Source: CAD feature listing. Evaluate the final solid. Frame: model axes, mm. A direction names the side the tool comes from. Give positions to 0.01 mm unless a question says otherwise; leave off trailing zeros. Write each loop counter-clockwise with the first axis right and the second up, starting at its lowest first coordinate (ties: lowest second). Pieces come first, ordered by that corner, then holes. Notation, with made-up numbers: (21.5, -40) - (44.5, -40) arc R6 ccw to (44.5, -33) - close; hole circle Ø9 at (82.25, 86.5). An arc over 180 degrees is marked (long way). One line per question, with ' | ' between items. Start each with the question number.
(1) Access query for faces 4 (the flat face through (-87, -68, 3)), 5 (the flat face through (-99.875, -71, 3)), 6 (the flat face through (23, 1, 6)). Directions: +Z, -Z, +X, -X, +Y, -Y. A direction counts if a zero-diameter tool reaches every point of the face in a straight line with its end or side. Return the directions, or none.
(2) Pin query (flat end, axial travel): pin 1 (3 mm diameter, centred on y = 14, z = 3, fed in from -X). Return the tip coordinate at first contact, or that it passes through.
(3) Section A-A, the plane y = 0. Return loops of the section in (x, z), plus the area to 3 significant figures.
(4) Section B-B, the plane x = 103. Return loops of the section in (y, z), plus the area to 3 significant figures.
(5) Section C-C, the plane x = -103. Return loops of the section in (y, z), plus the area to 3 significant figures.
(6) Draft query along Y for faces 1 (the flat face through (-2, 84.5, 3)), 2 (the flat face through (-109.5, 76, 3)), 3 (the flat face through (-106.125, -71, 3)). Return one class per face: +Y half, -Y half, draft (parallel to the pull), parting line (faces both ways), or undercut.
(7) Section D-D, the plane y = -78. Return loops of the section in (x, z).
(8) Ray query, line 1 (X direction, y = 78, z = 4.2); line 2 (Y direction, x = 103, z = 3.2); line 3 (Y direction, x = -103, z = 2.75). Return the intervals inside material, ascending. Write a range as [from, to].
Autodesk Inventor part; units mm, degrees
sketch "Sketch1" plane through (0, 0, 0) normal (0, 0, 1) x (1, 0, 0)
  line L0 (-109.5, 84.5) -> (109.5, 84.5)
  line L1 (109.5, 84.5) -> (109.5, -84.5)
  line L2 (109.5, -84.5) -> (-109.5, -84.5)
  line L3 (-109.5, -84.5) -> (-109.5, 84.5)
  point P0 (0, 84.5)
  point P1 (0, 0)
  point P2 (-109.5, 0)
  dimension "d0" = 219
  dimension "d1" = 169
extrude "Extrusion1" add sketch "Sketch1" along normal blind 6
sketch "Sketch2" plane through (0, 0, 6) normal (0, 0, 1) x (1, 0, 0)
  line L0 (-103, -84.5) -> (-103, -78) construction
  circle A0 centre (-103, -78) radius 3.25
  line L1 (-103, -78) -> (-103, -74) construction
  line L2 (-106.25, -68) -> (-99.75, -68)
  line L3 (-99.75, -68) -> (-99.75, -74)
  line L4 (-99.75, -74) -> (-106.25, -74)
  line L5 (-106.25, -74) -> (-106.25, -68)
  line L6 (-109.5, -84.5) -> (-103, -84.5) construction
  point P0 (0, 0)
  dimension "d38" = 6.5
  dimension "d39" = 6.5
  dimension "d44" = 4
  dimension "d45" = 6.5
  dimension "d46" = 6
  dimension "d58" = 6.5
extrude "Extrusion2" cut sketch "Sketch2" against normal blind 6 contours A0
mirror "Mirror3" about plane through (0, 0, 0) normal (1, 0, 0) of "Extrusion2"
mirror "Mirror7" about plane through (0, 0, 0) normal (0, 1, 0) of "Extrusion2", "Mirror3"
sketch "Sketch7" plane through (0, 0, 6) normal (0, 0, 1) x (1, 0, 0)
  line L0 (-109.5, 84.5) -> (-109.5, -84.5)
  line L1 (-109.5, 68) -> (-75, 68)
  line L2 (-75, 68) -> (-75, -68)
  line L3 (-75, -68) -> (-109.5, -68)
  line L4 (-109.5, -68) -> (-109.5, 68)
  point P0 (0, 0)
  point P1 (-109.5, 0)
  point P2 (-109.5, 0)
  dimension "d40" = 34.5
  dimension "d41" = 136
extrude "Extrusion6" cut sketch "Sketch7" against normal blind 10
sketch "Sketch8" plane through (0, 0, 6) normal (0, 0, 1) x (1, 0, 0)
  circle A0 centre (-103, -78) radius 3.25
  line L0 (-103, -78) -> (-103, -73.75) construction
  line L1 (-106.125, -68) -> (-99.875, -68)
  line L2 (-99.875, -68) -> (-99.875, -73.75)
  line L3 (-99.875, -73.75) -> (-106.125, -73.75)
  line L4 (-106.125, -73.75) -> (-106.125, -68)
  point P0 (0, 0)
  dimension "d47" = 4.25
  dimension "d48" = 6.25
  dimension "d49" = 5.75
extrude "Extrusion7" cut sketch "Sketch8" against normal blind 6 contours L1 L2 L3 L4
mirror "Mirror8" about plane through (0, 0, 0) normal (0, 1, 0) of "Extrusion7"
fillet "Fillet5" radius 1 12 edges at (-109.5, -84.5, 3) (109.5, -84.5, 3) (-75, -68, 3) (109.5, 84.5, 3) (-109.5, 84.5, 3) (-109.5, 68, 3) (-75, 68, 3) (-99.875, 68, 3) (-106.125, 68, 3) (-99.875, -68, 3) (-109.5, -68, 3) (-106.125, -68, 3)
sketch "Sketch9" plane through (0, 0, 6) normal (0, 0, 1) x (1, 0, 0)
  line L0 (-75, 44.5) -> (39, 44.5) construction
  line L1 (39, 44.5) -> (39, -44.5) construction
  line L2 (39, -44.5) -> (-75, -44.5) construction
  line L3 (-75, -44.5) -> (-75, 44.5) construction
  line L4 (-75, 67) -> (-75, -67)
  line L5 (39, 44.5) -> (-75, -44.5) construction
  circle A0 centre (0, 0) radius 19.25
  point P0 (-75, 0)
  point P1 (-75, 0)
  point P2 (-75, 0)
  dimension "d53" = 114
  dimension "d54" = 89
  dimension "d55" = 38.5
extrude "Extrusion8" cut sketch "Sketch9" against normal through all
equation "\"d7\" = d46"
properties part number "MDF_Top_Big_Mic" material "MDF Medium Density Fiberboard"
Check sheet entries:
1) face 4: +Z, -Z, -X | face 5: +Z, -Z | face 6: +Z, +X, -X, +Y, -Y
2) pin 1: x = -75
3) outline: (-75, 0) - (-19.25, 0) - (-19.25, 6) - (-75, 6) - close; (19.25, 0) - (109.5, 0) - (109.5, 6) - (19.25, 6) - close | area: 876 mm²
4) outline: (-84.5, 0) - (-81.25, 0) - (-81.25, 6) - (-84.5, 6) - close; (-74.75, 0) - (74.75, 0) - (74.75, 6) - (-74.75, 6) - close; (81.25, 0) - (84.5, 0) - (84.5, 6) - (81.25, 6) - close | area: 936 mm²
5) outline: (-84.5, 0) - (-81.25, 0) - (-81.25, 6) - (-84.5, 6) - close; (-74.75, 0) - (-73.75, 0) - (-73.75, 6) - (-74.75, 6) - close; (73.75, 0) - (74.75, 0) - (74.75, 6) - (73.75, 6) - close; (81.25, 0) - (84.5, 0) - (84.5, 6) - (81.25, 6) - close | area: 51.0 mm²
6) face 1: +Y half | face 2: draft | face 3: undercut
7) outline: (-109.5, 0) - (-106.25, 0) - (-106.25, 6) - (-109.5, 6) - close; (-99.75, 0) - (99.75, 0) - (99.75, 6) - (-99.75, 6) - close; (106.25, 0) - (109.5, 0) - (109.5, 6) - (106.25, 6) - close
8) line 1: [-109.5, -106.25], [-99.75, 99.75], [106.25, 109.5] | line 2: [-84.5, -81.25], [-74.75, 74.75], [81.25, 84.5] | line 3: [-84.5, -81.25], [-74.75, -73.75], [73.75, 74.75], [81.25, 84.5]
